Part model, mm, in its own coordinate system. A direction names the side the tool comes from. Round coordinates to 2 decimals unless told otherwise and drop trailing zeros. Write each loop counter-clockwise with the first axis right and the second up, starting at its lowest first coordinate (ties: lowest second). Pieces come first, ordered by that corner, then holes. Notation, with made-up numbers: (45, 83) -> (49, 83) arc R29 ccw to (49, 103) -> close; hole circle Ø1 at (49.25, 52.5). An arc over 180 degrees is marked (long way). Return JSON: item names as keys, results as strings. Group by question number.
(1) Tool access for faces 4 (the flat face through (-24.606, -3, 3)), 5 (the flat face through (0, 5, 3.175)), 6 (the flat face through (0, -17.145, 9)): list every direction of +Z, -Z, +X, -X, +Y, -Y with a clear straight run to the whole face (end or side of a thin tool).
(2) Saw through at B-B (z = 1). List the corners of the cut face in (x, y) (3 decimals), plus the area to 3 significant figures.
(3) Saw through at C-C (z = 6.25). List the corners of the cut face in (x, y) (3 decimals).
(4) Drill centre lines: L1, parallel to X at y = -14, z = 8; L2, parallel to Z at x = 9.5, y = 15.5 (3 decimals); L3, parallel to Y at x = -3, z = 8.5 (3 decimals). Where is each one in solid material? Low to high. Write a range as from..to.
(5) Drop flat-ended pins along their axis: pin 1 Ø2.5 at (x, z) = (-0.5, 7) entering from +Y (3 decimals); pin 2 Ø2 at (x, y) = (-15.875, -13.335) entering from -Z; pin 3 Ø3 at (x, z) = (16, 9.5) entering from -Y (3 decimals); pin 4 Ø1.5 at (x, y) = (-15.5, 4) entering from +Z (3 decimals). Give the stop position or say it passes through.
(6) Mould opens along X. For faces 1 (the cylindrical face through (-0.33, -17.66, 4.91)), 2 (the cylindrical face through (14.686, -13.283, 5.634)), 3 (the cylindrical face through (23.16, 17.52, 1.61)) say: +X half, -X half, draft (parallel to the pull), parting line (faces both ways), or undercut.
(7) Saw through at D-D (y = -1). List the corners of the cut face in (x, z) (3 decimals), plus the area to 3 significant figures.
from build123d import *

# Parameters (mm, degrees)
F0_W        = 49.2125
F0_H        = 38.1
F1_DEPTH    = 3.175
F2_W        = 49.2125
F2_H        = 7.62
F3_DEPTH    = 7.9375
F4_R        = 1.190625
F5_DEPTH    = 25.4
F6_T1_DEPTH = 49.2125
F7_R        = 5.08


# Not quite as in the source:
# - a fillet or chamfer that OpenCascade refuses, or shapes differently, is made with other operations: its cross-section is extruded or revolved along the edge and cut away or added


with BuildPart() as f1:
    # F0 (on Top) → F1 (new body)
    with BuildSketch(Plane.XY):
        Rectangle(F0_W, F0_H)
    extrude(amount=F1_DEPTH)

    # F2 (on face) → F3 (join)
    with BuildSketch(Plane.XY.offset(3.175)):
        with Locations((0, -13.335)):
            Rectangle(F2_W, F2_H)
    extrude(amount=F3_DEPTH)

    # F4 (on face) → F5 (cut)
    with BuildSketch(Plane.XY.offset(11.1125)):
        with Locations((-15.875, -13.335)):
            Circle(F4_R)
        with Locations((15.875, -13.335)):
            Circle(F4_R)
    extrude(amount=-F5_DEPTH, mode=Mode.SUBTRACT)

    # F6: fillet of radius 5.08 on 1 edges, made by hand

    # F6_s2 → F6_t1 (join)
    with BuildSketch(Plane.YZ.offset(-24.60625)):
        with BuildLine():
            ThreePointArc((-19.05, 3.175), (-17.6459498802, 4.9408692034), (-17.145, 7.140573729))
            Line((-17.145, 7.140573729), (-17.145, 3.175))
            Line((-17.145, 3.175), (-19.05, 3.175))
        make_face()
    extrude(amount=F6_T1_DEPTH)

    # F7
    f7_edges = [f1.edges().sort_by_distance(p)[0] for p in [
        (-24.60625, -19.05, 1.5875),
        (24.60625, -19.05, 1.5875),
        (24.60625, 19.05, 1.5875),
        (-24.60625, 19.05, 1.5875),
    ]]
    fillet(f7_edges, radius=F7_R)


solid = f1.part
Computed values:
{
 "1": {"face 4": "+Z, -Z, -X, +Y, -Y", "face 5": "+Z, +X, -X, +Y", "face 6": "+Z, +X, -X, -Y"},
 "2": {"outline": "(-24.606, -13.97) arc R5.08 ccw to (-19.526, -19.05) -> (19.526, -19.05) arc R5.08 ccw to (24.606, -13.97) -> (24.606, 13.97) arc R5.08 ccw to (19.526, 19.05) -> (-19.526, 19.05) arc R5.08 ccw to (-24.606, 13.97) -> close; hole circle Ø2.381 at (-15.875, -13.335); hole circle Ø2.381 at (15.875, -13.335)", "area": "1,840 mm2"},
 "3": {"outline": "(-24.606, -13.97) arc R5.08 ccw to (-23.428, -17.224) -> (23.428, -17.224) arc R5.08 ccw to (24.606, -13.97) -> (24.606, -9.525) -> (-24.606, -9.525) -> close; hole circle Ø2.381 at (-15.875, -13.335); hole circle Ø2.381 at (15.875, -13.335)"},
 "4": {"L1": "-24.61..-16.86, -14.89..14.89, 16.86..24.61", "L2": "0..3.175", "L3": "-17.145..-9.525"},
 "5": {"pin 1": "y = -9.525", "pin 2": "through", "pin 3": "y = -17.145", "pin 4": "z = 3.175"},
 "6": {"face 1": "draft", "face 2": "undercut", "face 3": "+X half"},
 "7": {"outline": "(-24.606, 0) -> (24.606, 0) -> (24.606, 3.175) -> (-24.606, 3.175) -> close", "area": "156 mm2"}
}
